from build123d import *

# Parameters (mm, degrees)
SKETCH2_W                    = 160
SKETCH2_H                    = 15
BASE_FLANGE1_DEPTH           = 2
EDGE_FLANGE1_STRIP_CUT_DEPTH = 15
EDGE_FLANGE1_DEPTH           = 15
EDGE_FLANGE2_STRIP_CUT_DEPTH = 15
EDGE_FLANGE2_DEPTH           = 15
EDGE_FLANGE3_STRIP_CUT_DEPTH = 15
EDGE_FLANGE3_DEPTH           = 15
EDGE_FLANGE4_STRIP_CUT_DEPTH = 15
EDGE_FLANGE4_DEPTH           = 15


# Sheet-metal steps are written as plain solids
with BuildPart() as part:
    # Sketch2 → Base-Flange1 (new body)
    with BuildSketch(Plane(origin=(48.130685362, 5.909705068, 0), x_dir=(0.014852136862004454, -0.1209609477998444, 0.9925461516413208), z_dir=(-0.9925461516413208, -0.12186934340515826, 0))):
        with Locations((80, -7.5)):
            Rectangle(SKETCH2_W, SKETCH2_H)
    extrude(amount=-BASE_FLANGE1_DEPTH)

    # Edge-Flange1 strip (across the edge) → Edge-Flange1 strip cut (cut)
    with BuildSketch(Plane(origin=(51.930191883, -8.623774192, -1.828040151), x_dir=(0.5091354036436435, -0.04382058195792874, 0.8595701817498632), z_dir=(-0.1209609477998443, 0.9851478631379957, 0.1218693434051582))):
        Polygon((-8.835731855, 2.791911088), (-0.6317, -1.944688912), (0.3683, -0.212638104), (-7.835731855, 4.523961896), align=None)
    extrude(amount=EDGE_FLANGE1_STRIP_CUT_DEPTH, mode=Mode.SUBTRACT)

    # Edge-Flange1 section (across the edge) → Edge-Flange1 (add)
    with BuildSketch(Plane(origin=(51.930191883, -8.623774192, -1.828040151), x_dir=(0.5091354036436435, -0.04382058195792874, 0.8595701817498632), z_dir=(-0.1209609477998443, 0.9851478631379957, 0.1218693434051582))):
        with BuildLine():
            Line((-2, 0.425276208), (-2, 33.845299462))
            Line((-2, 33.845299462), (0, 33.845299462))
            Line((0, 33.845299462), (0, 0.425276208))
            ThreePointArc((0, 0.425276208), (0.098685688, 0.056976208), (0.3683, -0.212638104))
            Line((0.3683, -0.212638104), (-0.6317, -1.944688912))
            ThreePointArc((-0.6317, -1.944688912), (-1.63336512, -0.943023792), (-2, 0.425276208))
        make_face()
    extrude(amount=EDGE_FLANGE1_DEPTH)

    # Edge-Flange2 strip (across the edge) → Edge-Flange2 strip cut (cut)
    with BuildSketch(Plane(origin=(77.938579558, 11.860163483, -18.515651229), x_dir=(-0.9925461516413208, -0.12186934340515852, 0), z_dir=(0.12096094779984468, -0.9851478631379958, -0.12186934340515816))):
        Polygon((-8.835731855, 2.791911088), (-0.6317, -1.944688912), (0.3683, -0.212638104), (-7.835731855, 4.523961896), align=None)
    extrude(amount=EDGE_FLANGE2_STRIP_CUT_DEPTH, mode=Mode.SUBTRACT)

    # Edge-Flange2 section (across the edge) → Edge-Flange2 (add)
    with BuildSketch(Plane(origin=(77.938579558, 11.860163483, -18.515651229), x_dir=(-0.9925461516413208, -0.12186934340515852, 0), z_dir=(0.12096094779984468, -0.9851478631379958, -0.12186934340515816))):
        with BuildLine():
            Line((-2, 0.425276208), (-2, 18.845299462))
            Line((-2, 18.845299462), (0, 18.845299462))
            Line((0, 18.845299462), (0, 0.425276208))
            ThreePointArc((0, 0.425276208), (0.098685688, 0.056976208), (0.3683, -0.212638104))
            Line((0.3683, -0.212638104), (-0.6317, -1.944688912))
            ThreePointArc((-0.6317, -1.944688912), (-1.63336512, -0.943023792), (-2, 0.425276208))
        make_face()
    extrude(amount=EDGE_FLANGE2_DEPTH)

    # Edge-Flange3 strip (across the edge) → Edge-Flange3 strip cut (cut)
    with BuildSketch(Plane(origin=(52.492119564, -13.200307893, 158.807384263), x_dir=(0.48341074799768535, 0.16568992536308802, -0.8595701817498632), z_dir=(0.12096094779984425, -0.9851478631379958, -0.1218693434051584))):
        Polygon((-8.835731855, 2.791911088), (-0.6317, -1.944688912), (0.3683, -0.212638104), (-7.835731855, 4.523961896), align=None)
    extrude(amount=EDGE_FLANGE3_STRIP_CUT_DEPTH, mode=Mode.SUBTRACT)

    # Edge-Flange3 section (across the edge) → Edge-Flange3 (add)
    with BuildSketch(Plane(origin=(52.492119564, -13.200307893, 158.807384263), x_dir=(0.48341074799768535, 0.16568992536308802, -0.8595701817498632), z_dir=(0.12096094779984425, -0.9851478631379958, -0.1218693434051584))):
        with BuildLine():
            Line((-2, 0.425276208), (-2, 33.845299462))
            Line((-2, 33.845299462), (0, 33.845299462))
            Line((0, 33.845299462), (0, 0.425276208))
            ThreePointArc((0, 0.425276208), (0.098685688, 0.056976208), (0.3683, -0.212638104))
            Line((0.3683, -0.212638104), (-0.6317, -1.944688912))
            ThreePointArc((-0.6317, -1.944688912), (-1.63336512, -0.943023792), (-2, 0.425276208))
        make_face()
    extrude(amount=EDGE_FLANGE3_DEPTH)

    # Edge-Flange4 strip (across the edge) → Edge-Flange4 strip cut (cut)
    with BuildSketch(Plane(origin=(82.683460004, -26.783786628, 175.494995341), x_dir=(-0.9925461516413208, -0.12186934340515758, 0), z_dir=(-0.12096094779984379, 0.9851478631379957, 0.12186934340515838))):
        Polygon((-8.835731855, 2.791911088), (-0.6317, -1.944688912), (0.3683, -0.212638104), (-7.835731855, 4.523961896), align=None)
    extrude(amount=EDGE_FLANGE4_STRIP_CUT_DEPTH, mode=Mode.SUBTRACT)

    # Edge-Flange4 section (across the edge) → Edge-Flange4 (add)
    with BuildSketch(Plane(origin=(82.683460004, -26.783786628, 175.494995341), x_dir=(-0.9925461516413208, -0.12186934340515758, 0), z_dir=(-0.12096094779984379, 0.9851478631379957, 0.12186934340515838))):
        with BuildLine():
            Line((-2, 0.425276208), (-2, 18.845299462))
            Line((-2, 18.845299462), (0, 18.845299462))
            Line((0, 18.845299462), (0, 0.425276208))
            ThreePointArc((0, 0.425276208), (0.098685688, 0.056976208), (0.3683, -0.212638104))
            Line((0.3683, -0.212638104), (-0.6317, -1.944688912))
            ThreePointArc((-0.6317, -1.944688912), (-1.63336512, -0.943023792), (-2, 0.425276208))
        make_face()
    extrude(amount=EDGE_FLANGE4_DEPTH)


solid = part.part
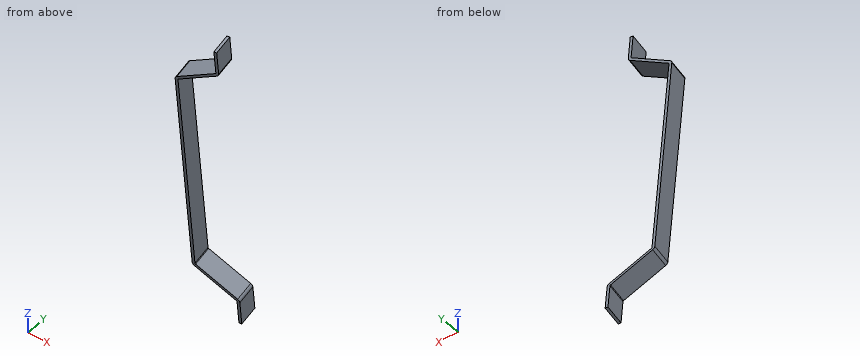
Verification items for the finished model (mm, model axes). Round coordinates to 2 decimals unless told otherwise and drop trailing zeros. Loops run counter-clockwise (first coordinate to the right, second up) from the corner with the lowest first, then second, coordinate; pieces in that order, holes last. Notation, with made-up numbers: (15.5, -20) - (63.5, -20) arc R34 ccw to (63.5, 19) - close; hole circle Ø3 at (48, -36). An arc over 180 degrees is marked (long way). Write item = value, one per line.
Q1. Sectioned sample at C-C on z = 90. Record the boundary of the cut face in (x, y), plus the area to 3 significant figures.
Here are the results:
outline = (49.48, -5.06) - (51.32, -20.06) - (53.3, -19.81) - (51.46, -4.81) - close
area = 30.2 mm^2
Q2. Material ranges on L1, parallel to X at y = -24, z = 170; L2, parallel to Z at x = 60, y = -20; L3, parallel to Z at x = 62, y = -5.5, recorded low to high.
Here are the results:
L1 = 71.96 to 76.1
L2 = 161.72 to 164.05
L3 = -9.96 to -7.63
Q3. Depth check by flat-ended pin: pin 1 (3 mm diameter, centred on x = 65, y = -14.5, fed in from +Z); pin 2 (12 mm diameter, centred on x = 67.5, y = 9, fed in from +Z); pin 3 (2 mm diameter, centred on x = 81, y = -22.5, fed in from +Z). Enter the tip coordinate at first touch or a pass-through.
Here are the results:
pin_1 = 168.81
pin_2 = -6.65
pin_3 = 176.03
Q4. Sectioned sample at A-A on x = 75.5. Record the boundary of the cut face in (y, z), plus the area to 3 significant figures.
Here are the results:
outline = (-27.16, 171.38) - (-26.88, 169.11) - (-12, 171.98) - (-12.29, 174.25) - close; (-4.03, -15.55) - (-3.75, -17.87) - (11.39, -17.1) - (11.1, -14.78) - close
area = 69.8 mm^2
Q5. Sectioned sample at B-B on z = 166. Record the boundary of the cut face in (x, y), plus the area to 3 significant figures.
Here are the results:
outline = (61.09, -13.03) - (66.1, -27.65) - (70.07, -27.16) - (65.06, -12.55) - close
area = 60.5 mm^2
